```python
from build123d import *

# Parameters (mm, degrees)
SKETCH3_W           = 37.35
SKETCH3_H           = 6
BOSS_EXTRUDE1_DEPTH = 4.75
SKETCH4_W           = 59.9
SKETCH4_H           = 39.5
SKETCH4_R           = 2.7
BOSS_EXTRUDE2_DEPTH = 6
CUT_EXTRUDE1_REACH  = 52.723
CHAMFER1_SIZE       = 1
CHAMFER2_SIZE       = 0.5


with BuildPart() as part:
    # Sketch3 → Boss-Extrude1 (new body)
    with BuildSketch(Plane(origin=(0, 0, 0), x_dir=(1, 0, 0), z_dir=(0, 1, 0))):
        with Locations((0, 3)):
            Rectangle(SKETCH3_W, SKETCH3_H)
    extrude(amount=BOSS_EXTRUDE1_DEPTH)

    # Sketch4 → Boss-Extrude2 (add)
    with BuildSketch(Plane(origin=(0, 0, 0), x_dir=(1, 0, 0), z_dir=(0, 1, 0))):
        with Locations((0, 19.75)):
            Rectangle(SKETCH4_W, SKETCH4_H)
        with Locations(Location((-24.95, 11.75, 0), (0, 0, 270))):
            Circle(SKETCH4_R, mode=Mode.SUBTRACT)
        with Locations(Location((-24.95, 27.75, 0), (0, 0, 270))):
            Circle(SKETCH4_R, mode=Mode.SUBTRACT)
        with Locations(Location((24.95, 11.75, 0), (0, 0, 270))):
            Circle(SKETCH4_R, mode=Mode.SUBTRACT)
        with Locations(Location((24.95, 27.75, 0), (0, 0, 270))):
            Circle(SKETCH4_R, mode=Mode.SUBTRACT)
    extrude(amount=-BOSS_EXTRUDE2_DEPTH)

    # Sketch5 → Cut-Extrude1 (cut, up to next)
    with BuildSketch(Plane.XZ.offset(6), mode=Mode.PRIVATE) as cut_extrude1_sk1:
        with BuildLine():
            Line((-17.87, -35.525), (-17.87, -39.5))
            Line((-17.87, -39.5), (13.536249219, -39.5))
            Line((13.536249219, -39.5), (13.536249219, -34.125))
            ThreePointArc((13.536249219, -34.125), (8.084468405, -28.650049236), (2.586446162, -34.078562046))
            ThreePointArc((2.586446162, -34.078562046), (2.342198533, -34.503972069), (1.851800837, -34.515833459))
            ThreePointArc((1.851800837, -34.515833459), (0.335489147, -34.21151821), (-1.099084421, -34.789279052))
            ThreePointArc((-1.099084421, -34.789279052), (-1.570217122, -34.872337403), (-1.895484475, -34.521529961))
            ThreePointArc((-1.895484475, -34.521529961), (-5.298347165, -31.486832634), (-9.38557377, -33.507585225))
            ThreePointArc((-9.38557377, -33.507585225), (-9.82, -33.760049669), (-10.25442623, -33.507585225))
            ThreePointArc((-10.25442623, -33.507585225), (-14.838500571, -31.585871726), (-17.87, -35.525))
        make_face()
    cut_extrude1_tool1 = extrude(cut_extrude1_sk1.sketch, amount=-CUT_EXTRUDE1_REACH, mode=Mode.PRIVATE) & part.part
    add(cut_extrude1_tool1.solids().sort_by_distance((-1.140343, -6, -35.39747))[0], mode=Mode.SUBTRACT)

    # Chamfer1
    chamfer1_edges = [part.edges().sort_by_distance(p)[0] for p in [
        (-29.95, -6, -19.75),
        (-29.95, -3, 0),
        (21.74312461, -6, -39.5),
        (-29.95, -3, -39.5),
        (29.95, -6, -19.75),
        (29.95, -3, -39.5),
        (0, -6, 0),
        (29.95, -3, 0),
        (-23.91, -6, -39.5),
    ]]
    chamfer(chamfer1_edges, length=CHAMFER1_SIZE)

    # Chamfer2
    chamfer2_edges = [part.edges().sort_by_distance(p)[0] for p in [
        (13.536249219, 0, -36.8125),
        (8.084468405, 0, -28.650049236),
        (2.342198533, 0, -34.503972069),
        (0.335489147, 0, -34.21151821),
        (-1.570217122, 0, -34.872337403),
        (-5.298347165, 0, -31.486832634),
        (-9.82, 0, -33.760049669),
        (-14.838500571, 0, -31.585871726),
        (-17.87, 0, -37.5125),
        (13.536249219, -6, -36.3125),
        (8.084468405, -6, -28.650049236),
        (2.342198533, -6, -34.503972069),
        (0.335489147, -6, -34.21151821),
        (-1.570217122, -6, -34.872337403),
        (-5.298347165, -6, -31.486832634),
        (-9.82, -6, -33.760049669),
        (-14.838500571, -6, -31.585871726),
        (-17.87, -6, -37.0125),
        (13.536249219, -2.5, -39.5),
        (-17.87, -2.5, -39.5),
    ]]
    chamfer(chamfer2_edges, length=CHAMFER2_SIZE - 0.0001)  # a hair under: the kernel refuses the full size


with BuildPart() as body_2:
    # Mirror1: mirrored copy
    add(part.part.mirror(Plane(origin=(0, -6, 0), x_dir=(0, 0, 1), z_dir=(0, -1, 0))))


solid = body_2.part
```
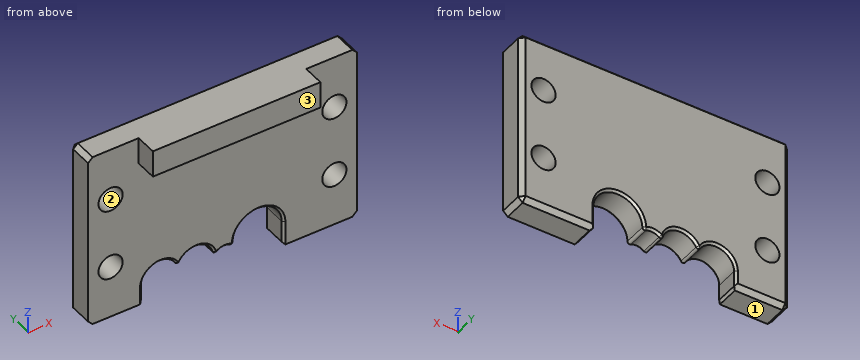
The listing builds one solid part. Answer for the finished solid, in the listing's coordinates (mm). Face numbers are marked on the shaded views. Coordinates: 2 decimals unless noted, no trailing zeros. Write each loop counter-clockwise with the first axis right and the second up, starting at its lowest first coordinate (ties: lowest second). Pieces come first, ordered by that corner, then holes. Notation, with made-up numbers: (7.25, -2) - (52.25, -2) arc R19 ccw to (52.25, 2) - close; hole circle Ø7 at (60.5, -31). An arc over 180 degrees is marked (long way). Return JSON: item names as keys, results as strings. Group by question number.
Q1. The part is cut by section D-D on z = -22. Write down the section's boundary in (x, y), and give its area (3 significant figures).
Q2. Find the intervals of material crossed by line 1 along X through (y, z) = (-8.35, -11.75); line 2 along X through (y, z) = (-7, -35.5); line 3 along Z through (x, y) = (26.5, -7.25), in increasing order. Write a range as [from, to].
Q3. The part is cut by section A-A on z = -11.75. Write down the section's boundary in (x, y), and give its area (3 significant figures).
Q4. The part is cut by section B-B on x = -24.95. Write down the section's boundary in (y, z).
Q5. Flat-ended cylindrical pins translate along their axes: pin 1 Ø3 at (x, y) = (-3, -8.5) entering from -Z; pin 2 Ø5 at (y, z) = (-15, -3.5) entering from -X (3 decimals); pin 3 Ø7 at (x, z) = (24.95, -27.75) entering from -Y. Find the tip coordinate at first contact, or state that the pin passes through.
Q6. For a pull along Z with two mould halves and no side action, classify the marked faces 1, 2 and 3 as +Z half, -Z half, draft (parallel to the pull), parting line (faces both ways), or undercut.
Q7. The part is cut by section C-C on y = -10. Write down the section's boundary in (x, z) (3 decimals).
Evaluation:
{
 "1": {"outline": "(-29.95, -12) - (29.95, -12) - (29.95, -7) - (28.95, -6) - (-28.95, -6) - (-29.95, -7) - close", "area": "358 mm2"},
 "2": {"line 1": "x = [-29.95, -27.65], [-22.25, 22.25], [27.65, 29.95]", "line 2": "x = [-29.95, -17.87], [13.54, 29.95]", "line 3": "z = [-39.5, -29.96], [-25.54, -13.96], [-9.54, 0]"},
 "3": {"outline": "(-29.95, -12) - (-27.65, -12) - (-27.65, -6) - (-28.95, -6) - (-29.95, -7) - close; (-22.25, -12) - (22.25, -12) - (22.25, -6) - (-22.25, -6) - close; (27.65, -12) - (29.95, -12) - (29.95, -7) - (28.95, -6) - (27.65, -6) - close", "area": "294 mm2"},
 "4": {"outline": "(-12, -39.5) - (-7, -39.5) - (-6, -38.5) - (-6, -30.45) - (-12, -30.45) - close; (-12, -25.05) - (-6, -25.05) - (-6, -14.45) - (-12, -14.45) - close; (-12, -9.05) - (-6, -9.05) - (-6, -1) - (-7, 0) - (-12, 0) - close"},
 "5": {"pin 1": "stops at z = -34.89", "pin 2": "stops at x = -18.675", "pin 3": "stops at y = -12"},
 "6": {"face 1": "-Z half", "face 2": "undercut", "face 3": "draft"},
 "7": {"outline": "(-29.95, -38.5) - (-28.95, -39.5) - (-18.37, -39.5) - (-17.87, -39) - (-17.87, -35.525) arc R4.075 cw to (-10.254, -33.508) arc R0.5 ccw to (-9.386, -33.508) arc R4.075 cw to (-1.895, -34.522) arc R0.5 ccw to (-1.099, -34.789) arc R2.7 cw to (1.852, -34.516) arc R0.5 ccw to (2.586, -34.079) arc R5.475 cw to (13.536, -34.125) - (13.536, -39) - (14.036, -39.5) - (28.95, -39.5) - (29.95, -38.5) - (29.95, -1) - (28.95, 0) - (-28.95, 0) - (-29.95, -1) - close; hole circle Ø5.4 at (-24.95, -27.75); hole circle Ø5.4 at (-24.95, -11.75); hole circle Ø5.4 at (24.95, -27.75); hole circle Ø5.4 at (24.95, -11.75)"}
}
